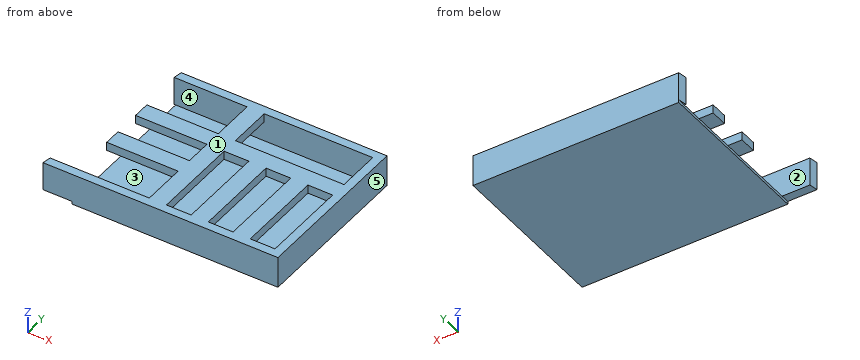
from build123d import *

# Parameters (mm, degrees)
F0_W     = 457.2
F0_H     = 368.3
F1_DEPTH = 6.35
F2_W     = 19.05
F2_H     = 330.2
F3_DEPTH = 63.5
F4_W     = 158.75
F4_H     = 38.1
F4_W_2   = 55.0164
F4_W_3   = 55.0418
F5_DEPTH = 19.05


with BuildPart() as f1:
    # F0 (on Top) → F1 (new body)
    with BuildSketch(Plane.XY):
        with Locations((228.6, 184.15)):
            Rectangle(F0_W, F0_H)
    extrude(amount=F1_DEPTH)

    # F2 (on face) → F3 (join)
    with BuildSketch(Plane.XY.offset(6.35)):
        Polygon((-61.582198, 19.05), (-64.941227, 0), (0, 0), (0, 19.05), align=None)
        Polygon((0, 19.05), (0, 0), (457.2, 0), (457.2, 19.05), (438.15, 19.05), align=None)
        with Locations((447.675, 184.15)):
            Rectangle(F2_W, F2_H)
        Polygon((0, 368.3), (0, 349.25), (438.15, 349.25), (457.2, 349.25), (457.2, 368.3), align=None)
        Polygon((-3.359029, 349.25), (0, 349.25), (0, 368.3), align=None)
    extrude(amount=F3_DEPTH)

    # F4 (on face) → F5 (join)
    with BuildSketch(Plane.XY.offset(69.85)):
        with Locations((79.375, 232.8418)):
            Rectangle(F4_W, F4_H)
        Polygon((196.85, 213.7918), (196.85, 251.8918), (196.85, 349.25), (158.75, 349.25), (158.75, 251.8918), (158.75, 213.7918), (158.75, 154.5336), (158.75, 116.4336), (158.75, 19.05), (196.85, 19.05), align=None)
        with Locations((224.3582, 232.8418)):
            Rectangle(F4_W_2, F4_H)
        Polygon((289.9664, 19.05), (289.9664, 213.7918), (289.9664, 251.8918), (251.8664, 251.8918), (251.8664, 213.7918), (251.8664, 19.05), align=None)
        with Locations((317.4873, 232.8418)):
            Rectangle(F4_W_3, F4_H)
        Polygon((345.0082, 19.05), (383.1082, 19.05), (383.1082, 213.7918), (383.1082, 251.8918), (345.0082, 251.8918), (345.0082, 213.7918), align=None)
        with Locations((410.6291, 232.8418)):
            Rectangle(F4_W_3, F4_H)
        with Locations((79.375, 135.4836)):
            Rectangle(F4_W, F4_H)
    extrude(amount=-F5_DEPTH)


solid = f1.part
Can you work these out from the model? Positions are in its coordinate system, mm. Face numbers are marked on the shaded views. A direction names the side the tool comes from. Give positions to 0.01 mm unless a question says otherwise; leave off trailing zeros. Order: outer loops, then holes, each group sorted by start corner. A loop starts at its lowest first (then second) coordinate and runs counter-clockwise, first axis right, second up. Notation, with made-up numbers: M 3.25,4 L 12.25,4 A21 cw 12.25,16 Z; hole C 62,14 d9. An arc over 180 degrees is marked long. Use a Markdown table: item, result. Add a question column.
Item 1: Suppose I cut it at B-B (x = 395). List the corners of the cut face in (y, z) for me.
Item 2: For the marked faces 1 and 2, which set-ups out of +Z, -Z, +X, -X, +Y, -Y let a thin tool reach every point of the face, with its end or its side?
Item 3: Suppose I cut it at D-D (x = 87.5). List the corners of the cut face in (y, z) for me.
Item 4: Will these pins go through, and if not, where does the flat tip stop? pin 1 (10 mm diameter, centred on y = 170.5, z = 17, fed in from -X); pin 2 (15 mm diameter, centred on y = 99.5, z = 58.5, fed in from -X); pin 3 (9.5 mm diameter, centred on y = 135.5, z = 63, fed in from -X).
Item 5: We'd pull the mould along X, two halves only. Please class the marked faces 3, 4 and 5: +X half, -X half, draft (parallel to the pull), parting line (faces both ways), or undercut.
Item 6: Suppose I cut it at A-A (y = 298). List the corners of the cut face in (x, z) for me.
Item 7: Suppose I cut it at C-C (y = 132). List the corners of the cut face in (x, z) for me.
Item 8: If I drill on L1, parallel to X at y = 146.5, z = 64; L2, parallel to Y at x = 83, z = 11; L3, parallel to Y at x = 76, z = 65.5, over which ranges is the centre line in solid material (lowest first)? Write a range as [from, to].
Answer sheet:
| question | item | result |
|---|---|---|
| 1 | outline | M 0,0 L 368.3,0 L 368.3,69.85 L 349.25,69.85 L 349.25,6.35 L 19.05,6.35 L 19.05,69.85 L 0,69.85 Z; M 213.79,50.8 L 251.89,50.8 L 251.89,69.85 L 213.79,69.85 Z |
| 2 | face 1 | +Z, +X, -X, +Y, -Y |
| 2 | face 2 | none |
| 3 | outline | M 0,0 L 368.3,0 L 368.3,69.85 L 349.25,69.85 L 349.25,6.35 L 19.05,6.35 L 19.05,69.85 L 0,69.85 Z; M 116.43,50.8 L 154.53,50.8 L 154.53,69.85 L 116.43,69.85 Z; M 213.79,50.8 L 251.89,50.8 L 251.89,69.85 L 213.79,69.85 Z |
| 4 | pin 1 | stops at x = 438.15 |
| 4 | pin 2 | stops at x = 158.75 |
| 4 | pin 3 | stops at x = 0 |
| 5 | face 3 | draft |
| 5 | face 4 | undercut |
| 5 | face 5 | +X half |
| 6 | outline | M 0,0 L 457.2,0 L 457.2,69.85 L 438.15,69.85 L 438.15,6.35 L 0,6.35 Z; M 158.75,50.8 L 196.85,50.8 L 196.85,69.85 L 158.75,69.85 Z |
| 7 | outline | M 0,0 L 457.2,0 L 457.2,69.85 L 438.15,69.85 L 438.15,6.35 L 0,6.35 Z; M 0,50.8 L 196.85,50.8 L 196.85,69.85 L 0,69.85 Z; M 251.87,50.8 L 289.97,50.8 L 289.97,69.85 L 251.87,69.85 Z; M 345.01,50.8 L 383.11,50.8 L 383.11,69.85 L 345.01,69.85 Z |
| 8 | L1 | x = [0, 196.85], [251.87, 289.97], [345.01, 383.11], [438.15, 457.2] |
| 8 | L2 | y = [0, 19.05], [349.25, 368.3] |
| 8 | L3 | y = [0, 19.05], [116.43, 154.53], [213.79, 251.89], [349.25, 368.3] |
